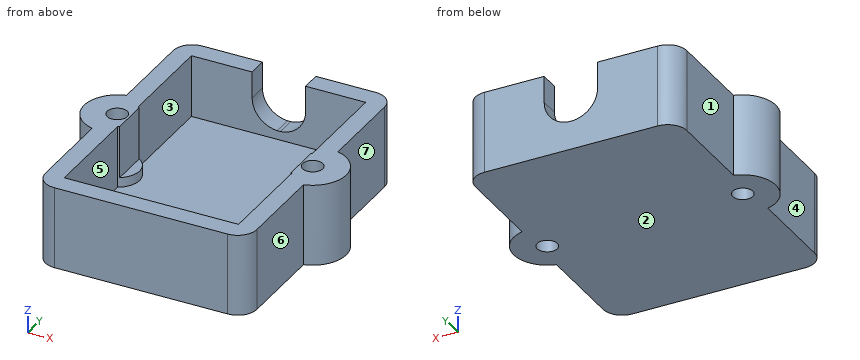
from build123d import *

# Parameters (mm, degrees)
BOSS_EXTRUDE2_DEPTH = 8.595
CUT_EXTRUDE3_REACH  = 34.514
SKETCH5_R           = 1.06
CUT_EXTRUDE4_DEPTH  = 6.525
CUT_EXTRUDE2_REACH  = 35.545
SKETCH7_W           = 18
SKETCH7_H           = 24.65
CUT_EXTRUDE6_DEPTH  = 5.5


with BuildPart() as part:
    # Sketch1 → Boss-Extrude2 (new body)
    with BuildSketch(Plane.XY):
        with BuildLine():
            Line((-11.11, 0.816412174), (-11.11, 10.090766215))
            ThreePointArc((-11.11, 10.090766215), (-13.747229408, 13.5), (-11.11, 16.909233785))
            Line((-11.11, 16.909233785), (-11.11, 26.183587826))
            ThreePointArc((-11.11, 26.183587826), (-10.524213562, 27.597801388), (-9.11, 28.183587826))
            Line((-9.11, 28.183587826), (9.06, 28.183587826))
            ThreePointArc((9.06, 28.183587826), (10.474213562, 27.597801388), (11.06, 26.183587826))
            Line((11.06, 26.183587826), (11.06, 16.909233785))
            ThreePointArc((11.06, 16.909233785), (13.735, 13.5), (11.06, 10.090766215))
            Line((11.06, 10.090766215), (11.06, 0.816412174))
            ThreePointArc((11.06, 0.816412174), (10.474213562, -0.597801388), (9.06, -1.183587826))
            Line((9.06, -1.183587826), (-9.11, -1.183587826))
            ThreePointArc((-9.11, -1.183587826), (-10.524213562, -0.597801388), (-11.11, 0.816412174))
        make_face()
    extrude(amount=BOSS_EXTRUDE2_DEPTH)

    # Sketch5 → Cut-Extrude3 (cut, up to next)
    with BuildSketch(Plane.XY.offset(8.595), mode=Mode.PRIVATE) as cut_extrude3_sk1:
        with Locations((-10.275, 13.5)):
            Circle(SKETCH5_R)
    cut_extrude3_tool1 = extrude(cut_extrude3_sk1.sketch, amount=-CUT_EXTRUDE3_REACH, mode=Mode.PRIVATE) & part.part
    # Sketch5 → Cut-Extrude3 (cut, up to next)
    with BuildSketch(Plane.XY.offset(8.595), mode=Mode.PRIVATE) as cut_extrude3_sk2:
        with Locations(Location((10.225, 13.5, 0), (0, 0, 180))):
            Circle(SKETCH5_R)
    cut_extrude3_tool2 = extrude(cut_extrude3_sk2.sketch, amount=-CUT_EXTRUDE3_REACH, mode=Mode.PRIVATE) & part.part
    add(cut_extrude3_tool1.solids().sort_by_distance((-10.275, 13.5, 8.595))[0], mode=Mode.SUBTRACT)
    add(cut_extrude3_tool2.solids().sort_by_distance((10.225, 13.5, 8.595))[0], mode=Mode.SUBTRACT)

    # Sketch2 → Cut-Extrude4 (cut)
    with BuildSketch(Plane.XY.offset(8.595)):
        with BuildLine():
            Line((-9.1625, 15.528570386), (-9.1625, 26.136412174))
            Line((-9.1625, 26.136412174), (9.1125, 26.136412174))
            Line((9.1125, 26.136412174), (9.1125, 15.528570386))
            ThreePointArc((9.1125, 15.528570386), (7.885020948, 13.5), (9.1125, 11.471429614))
            Line((9.1125, 11.471429614), (9.1125, 0.861412174))
            Line((9.1125, 0.861412174), (-9.1625, 0.861412174))
            Line((-9.1625, 0.861412174), (-9.1625, 11.471429614))
            ThreePointArc((-9.1625, 11.471429614), (-7.935020948, 13.5), (-9.1625, 15.528570386))
        make_face()
    extrude(amount=-CUT_EXTRUDE4_DEPTH, mode=Mode.SUBTRACT)

    # Sketch3 → Cut-Extrude2 (cut, up to next)
    with BuildSketch(Plane(origin=(0, 28.183587826, 0), x_dir=(1, 0, 0), z_dir=(0, 1, 0)), mode=Mode.PRIVATE) as cut_extrude2_sk1:
        with BuildLine():
            Line((0.167257287, -3.005), (-0.167257287, -3.005))
            ThreePointArc((-0.167257287, -3.005), (-2.038175704, -3.880145891), (-2.8, -5.8))
            Line((-2.8, -5.8), (-2.8, -8.595))
            Line((-2.8, -8.595), (-0.167257287, -8.595))
            Line((-0.167257287, -8.595), (0.167257287, -8.595))
            Line((0.167257287, -8.595), (2.8, -8.595))
            Line((2.8, -8.595), (2.8, -5.8))
            ThreePointArc((2.8, -5.8), (2.038175704, -3.880145891), (0.167257287, -3.005))
        make_face()
    cut_extrude2_tool1 = extrude(cut_extrude2_sk1.sketch, amount=-CUT_EXTRUDE2_REACH, mode=Mode.PRIVATE) & part.part
    add(cut_extrude2_tool1.solids().sort_by_distance((0, 28.183588, 6.058962))[0], mode=Mode.SUBTRACT)

    # Sketch7 → Cut-Extrude6 (cut)
    with BuildSketch(Plane.XY.offset(8.595)):
        with Locations((0, 13.548319596)):
            Rectangle(SKETCH7_W, SKETCH7_H)
    extrude(amount=-CUT_EXTRUDE6_DEPTH, mode=Mode.SUBTRACT)


solid = part.part
Design review of the part built by this model. Coordinates are the model's own, in mm. Face numbers are marked on the shaded views. A direction names the side the tool comes from. Give positions to 0.01 mm unless a question says otherwise; leave off trailing zeros. Order: outer loops, then holes, each group sorted by start corner. A loop starts at its lowest first (then second) coordinate and runs counter-clockwise, first axis right, second up. Notation, with made-up numbers: (9, -32.75) - (41, -32.75) arc R11 cw to (41, -19.75) - close; hole circle Ø5 at (50, -33.5). An arc over 180 degrees is marked (long way). Use CSV: the item, a comma, the result in double quotes. Start each with the question number.
Q1. Machinability: for the marked faces 4, 5, 6 and 7, which of the approach directions +Z, -Z, +X, -X, +Y, -Y give a long, thin tool a straight path to every point of the face, cutting with its end or side? Answer none if there is none.
Q2. Draft analysis for pull direction X (two halves, no side actions). For the marked faces 1, 2 and 3, state which applies: pulls with the +X half, pulls with the -X half, needs draft (parallel to the pull), parting line crosses it, or undercut.
Q3. Take a section at A-A (y = 13.5). State the section outline as (x, z) points (3 decimals).
Q4. Take a section at B-B (z = 7.5). Count the separate pieces of the cut face and the enclosed holes in it, and give its area (3 significant figures).
Q5. For line 1 (Y direction, x = -6.5, z = 5); line 2 (X direction, y = 22.75, z = 3); line 3 (Z direction, x = 3.75, y = 17.5), list the stretches that pass through material, from the lowest coordinate up.
Q6. For P1, Ø1.5, axis at y = 5, z = 1, coming from the +X side; P2, Ø1.9, axis at x = 10.225, y = 13.5, coming from the -Z side; P3, Ø1.2, axis at y = 14.5, z = 6.5, coming from the -X side; P4, Ø0.5, axis at x = -8.5, y = 13, coming from the +Z side (3 decimals), all flat-tipped, find the tip position at first contact; note any pin that passes through.
Q7. Take a section at D-D (y = 25.25). State the section outline as (x, z) points (1 decimal), and give its area (3 significant figures).
Q8. Take a section at C-C (x = -7.5). State the section outline as (y, z) points (3 decimals), and give its area (3 significant figures).
Calculated:
1,face 4,"+Z, -Z, -X, -Y"
1,face 5,"+Z"
1,face 6,"+Z, -Z, +X, -Y"
1,face 7,"+Z, -Z, +X, +Y"
2,face 1,"pulls with the -X half"
2,face 2,"needs draft"
2,face 3,"undercut"
3,outline,"(-13.747, 0) - (-11.335, 0) - (-11.335, 8.595) - (-13.747, 8.595) - close; (-9.215, 0) - (9.165, 0) - (9.165, 8.595) - (9, 8.595) - (9, 3.095) - (7.885, 3.095) - (7.885, 2.07) - (-7.935, 2.07) - (-7.935, 3.095) - (-9, 3.095) - (-9, 8.595) - (-9.215, 8.595) - close; (11.285, 0) - (13.735, 0) - (13.735, 8.595) - (11.285, 8.595) - close"
4,separate pieces,"1"
4,enclosed holes,"2"
4,area,"195 mm²"
5,line 1,"y = -1.18 to 0.86, 26.14 to 28.18"
5,line 2,"x = -11.11 to -9.16, 9.11 to 11.06"
5,line 3,"z = 0 to 2.07"
6,P1,"stops at x = 11.06"
6,P2,"passes through"
6,P3,"stops at x = -13.72"
6,P4,"stops at z = 3.095"
7,outline,"(-11.1, 0) - (11.1, 0) - (11.1, 8.6) - (9.1, 8.6) - (9.1, 2.1) - (-9.2, 2.1) - (-9.2, 8.6) - (-11.1, 8.6) - close"
7,area,"71.3 mm²"
8,outline,"(-1.184, 0) - (28.184, 0) - (28.184, 8.595) - (26.136, 8.595) - (26.136, 2.07) - (0.861, 2.07) - (0.861, 8.595) - (-1.184, 8.595) - close"
8,area,"87.5 mm²"
